```python
from build123d import *

# Parameters (mm, degrees)
BOSS_EXTRUDE1_DEPTH = 6
SKETCH3_R           = 5
CUT_EXTRUDE1_DEPTH  = 262.076617107
SKETCH4_R           = 5
CUT_EXTRUDE2_DEPTH  = 262.076617107
CUT_EXTRUDE5_DEPTH  = 262.076617107
FILLET5_R           = 5
FILLET6_R           = 5
SKETCH9_W           = 500
SKETCH9_H           = 10
BOSS_EXTRUDE2_DEPTH = 6


with BuildPart() as part:
    # Sketch1 → Boss-Extrude1 (new body)
    with BuildSketch(Plane.XY):
        with BuildLine():
            Line((-250, -55), (-250, 3.178280867))
            Line((-250, 3.178280867), (-250, 55))
            ThreePointArc((-250, 55), (-244.142135624, 69.142135624), (-230, 75))
            Line((-230, 75), (-220, 75))
            Line((-220, 75), (-164.330865428, 75))
            Line((-164.330865428, 75), (-60, 75))
            ThreePointArc((-60, 75), (-52.928932188, 72.071067812), (-50, 65))
            Line((-50, 65), (-50, 20))
            ThreePointArc((-50, 20), (-48.100925873, 14.1369803), (-43.125, 10.500822404))
            ThreePointArc((-43.125, 10.500822404), (-39.437786703, 8.32242004), (-37, 4.801315846))
            ThreePointArc((-37, 4.801315846), (-22.271648276, -13.226099426), (0, -20))
            Line((0, -20), (0, -40))
            Line((0, -40), (0, -65))
            Line((0, -65), (0, -75))
            Line((0, -75), (-230, -75))
            ThreePointArc((-230, -75), (-244.142135624, -69.142135624), (-250, -55))
        make_face()
    boss_extrude1 = extrude(amount=BOSS_EXTRUDE1_DEPTH)

    # Mirror1: Boss-Extrude1 across plane
    add(boss_extrude1.mirror(Plane(origin=(0, -20, 6), x_dir=(0, 0, 1), z_dir=(-1, 0, 0))))

    # Sketch3 → Cut-Extrude1 (cut, through all)
    with BuildSketch(Plane.XY.offset(6)):
        with Locations((110, 55)):
            Circle(SKETCH3_R)
        with Locations((200, 55)):
            Circle(SKETCH3_R)
        with Locations((-110, 55)):
            Circle(SKETCH3_R)
        with Locations((-200, 55)):
            Circle(SKETCH3_R)
    extrude(amount=-CUT_EXTRUDE1_DEPTH, mode=Mode.SUBTRACT)

    # Sketch4 → Cut-Extrude2 (cut, through all)
    with BuildSketch(Plane.XY.offset(6)):
        with BuildLine():
            Line((-70, -55), (-70, 25))
            ThreePointArc((-70, 25), (-72.928932188, 32.071067812), (-80, 35))
            Line((-80, 35), (-110, 35))
            ThreePointArc((-110, 35), (-113.535533906, 33.535533906), (-115, 30))
            Line((-115, 30), (-115, 25))
            ThreePointArc((-115, 25), (-115.614239502, 21.549275456), (-117.381499976, 18.522465177))
            ThreePointArc((-117.381499976, 18.522465177), (-117.5115076, 18.372596167), (-117.644462896, 18.225335882))
            ThreePointArc((-117.644462896, 18.225335882), (-122.017250069, 15.45520022), (-127.189262676, 15.242585951))
            ThreePointArc((-127.189262676, 15.242585951), (-127.232362089, 15.252356208), (-127.275417902, 15.262316838))
            ThreePointArc((-127.275417902, 15.262316838), (-131.839411289, 17.704627959), (-134.570789944, 22.101728126))
            ThreePointArc((-134.570789944, 22.101728126), (-134.892115533, 23.535059632), (-135, 25))
            Line((-135, 25), (-135, 30))
            ThreePointArc((-135, 30), (-136.464466094, 33.535533906), (-140, 35))
            Line((-140, 35), (-215, 35))
            ThreePointArc((-215, 35), (-218.535533906, 33.535533906), (-220, 30))
            Line((-220, 30), (-220, 25))
            ThreePointArc((-220, 25), (-220.586588267, 21.625436392), (-222.277535909, 18.646768667))
            ThreePointArc((-222.277535909, 18.646768667), (-226.488765584, 15.636708224), (-231.640827685, 15.135534251))
            ThreePointArc((-231.640827685, 15.135534251), (-237.629163678, 18.535028107), (-240, 25))
            Line((-240, 25), (-240, -55))
            ThreePointArc((-240, -55), (-237.071067812, -62.071067812), (-230, -65))
            Line((-230, -65), (-210, -65))
            Line((-210, -65), (-190, -65))
            Line((-190, -65), (-110, -65))
            Line((-110, -65), (-90, -65))
            Line((-90, -65), (-80, -65))
            ThreePointArc((-80, -65), (-72.928932188, -62.071067812), (-70, -55))
        make_face()
        with Locations((-230, 25)):
            Circle(SKETCH4_R)
        with Locations((-125, 25)):
            Circle(SKETCH4_R)
    cut_extrude2 = extrude(amount=-CUT_EXTRUDE2_DEPTH, mode=Mode.SUBTRACT)

    # Sketch8 → Cut-Extrude5 (cut, through all)
    with BuildSketch(Plane.XY.offset(6)):
        with BuildLine():
            Line((-60, 0), (-60, -65))
            Line((-60, -65), (60, -65))
            Line((60, -65), (60, 0))
            ThreePointArc((60, 0), (57.236067977, 4.472135955), (52, 4))
            ThreePointArc((52, 4), (49.247332505, 2.266223145), (46.25, 1.001644808))
            ThreePointArc((46.25, 1.001644808), (0, -30), (-46.25, 1.001644808))
            ThreePointArc((-46.25, 1.001644808), (-49.247332505, 2.266223145), (-52, 4))
            ThreePointArc((-52, 4), (-57.236067977, 4.472135955), (-60, 0))
        make_face()
    extrude(amount=-CUT_EXTRUDE5_DEPTH, mode=Mode.SUBTRACT)

    # Fillet5
    fillet5_edges = [part.edges().sort_by_distance(p)[0] for p in [
        (-60, -65, 3),
    ]]
    fillet(fillet5_edges, radius=FILLET5_R)

    # Fillet6
    fillet6_edges = [part.edges().sort_by_distance(p)[0] for p in [
        (60, -65, 3),
    ]]
    fillet(fillet6_edges, radius=FILLET6_R)

    # Mirror2: Cut-Extrude2 across plane
    add(cut_extrude2.mirror(Plane(origin=(0, 0, 0), x_dir=(0, 0, 1), z_dir=(1, 0, 0))), mode=Mode.SUBTRACT)

    # Sketch9 → Boss-Extrude2 (add)
    with BuildSketch(Plane.XY.offset(6)):
        with Locations((0, -25)):
            Rectangle(SKETCH9_W, SKETCH9_H)
    extrude(amount=-BOSS_EXTRUDE2_DEPTH)


solid = part.part
```
For this review, take the finished solid that the model builds, in its own axes (mm). A direction names the side the tool comes from. Coordinates: 2 decimals unless noted, no trailing zeros. Loops run counter-clockwise (first coordinate to the right, second up) from the corner with the lowest first, then second, coordinate; pieces in that order, holes last.
1. For faces 5 (the cylindrical face through (53.01, 72.15, 2.96)), 6 (the cylindrical face through (-237.15, -61.99, 3.04)), 7 (the cylindrical face through (244.297, 68.986, 2.958)), list the 3-axis set-ups (+Z, -Z, +X, -X, +Y, -Y) from which the entire face can be reached by the end or side of a thin tool; tool diameter is ignored.
2. Add section C-C, the plane y = -49. Give the boundary of the cut face in (x, z), then the cut area to 3 significant figures.
3. Add section A-A, the plane x = 165. Give the boundary of the cut face in (y, z).
4. Add section D-D, the plane z = 2.5. Count the separate pieces of the cut face and the enclosed holes in it, then the cut area to 3 significant figures.
5. For line 1 (Y direction, x = -206, z = 4.55); line 2 (Y direction, x = 124.5, z = 1.4); line 3 (Y direction, x = 110, z = 2.1), list the stretches that pass through material, from the lowest coordinate up.
6. Mouldability with a two-part tool opening along Y and no side actions: class faces 1 (the cylindrical face through (72.85, 31.99, 3.04)), 2 (the cylindrical face through (225.23, 26.5, 3.04)), 3 (the cylindrical face through (-244.297, 68.986, 2.958)), 4 (the cylindrical face through (-243.986, -69.297, 2.958)) as +Y half, -Y half, draft (parallel to the pull), parting line (faces both ways), or undercut.
7. Add section B-B, the plane x = -200. Give the boundary of the cut face in (y, z), then the cut area to 3 significant figures.
Result:
1. face 5: +Z, -Z, +Y
1. face 6: +Z, -Z
1. face 7: +Z, -Z, +X, +Y
2. outline: (-250, 0) - (-240, 0) - (-240, 6) - (-250, 6) - close; (-70, 0) - (-60, 0) - (-60, 6) - (-70, 6) - close; (60, 0) - (70, 0) - (70, 6) - (60, 6) - close; (240, 0) - (250, 0) - (250, 6) - (240, 6) - close
2. area: 240 mm2
3. outline: (-75, 0) - (-65, 0) - (-65, 6) - (-75, 6) - close; (-30, 0) - (-20, 0) - (-20, 6) - (-30, 6) - close; (35, 0) - (75, 0) - (75, 6) - (35, 6) - close
4. separate pieces: 1
4. enclosed holes: 15
4. area: 31,700 mm2
5. line 1: y = -75 to -65, -30 to -20, 35 to 75
5. line 2: y = -75 to -65, -30 to -20, 15.01 to 20.03, 29.97 to 75
5. line 3: y = -75 to -65, -30 to -20, 35 to 50, 60 to 75
6. face 1: undercut
6. face 2: undercut
6. face 3: +Y half
6. face 4: -Y half
7. outline: (-75, 0) - (-65, 0) - (-65, 6) - (-75, 6) - close; (-30, 0) - (-20, 0) - (-20, 6) - (-30, 6) - close; (35, 0) - (50, 0) - (50, 6) - (35, 6) - close; (60, 0) - (75, 0) - (75, 6) - (60, 6) - close
7. area: 300 mm2
